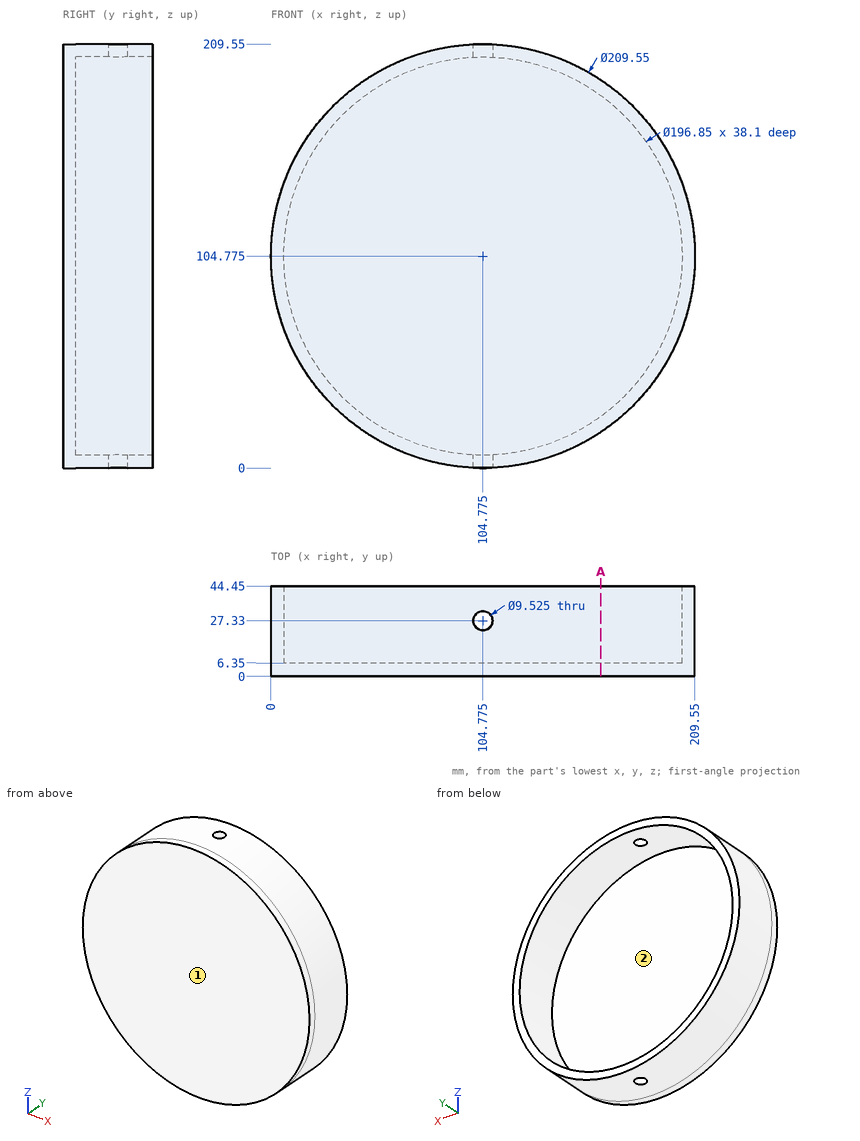
Part print with two shaded views. Sizes in mm from the minimum x, y, z corner. Give positions to 0.01 mm unless a question says otherwise; leave off trailing zeros. Order: outer loops, then holes, each group sorted by start corner. A loop starts at its lowest first (then second) coordinate and runs counter-clockwise, first axis right, second up. Notation, with made-up numbers: M -4.75,-21.75 L 11.25,-21.75 A14 cw 11.25,-9.75 Z; hole C 16.5,85.5 d10. An arc over 180 degrees is marked long. Write item = value, one per line.
Q1. Drill centre lines: line 1 (X direction, y = 26, z = 105); line 2 (Y direction, x = 145, z = 141); line 3 (Z direction, x = 31.5, y = 10.5) (1 decimal). Where is each one in solid material? Low to high. Write a range as [from, to].
Derived:
line_1 = [0, 6.35], [203.2, 209.55]
line_2 = [0, 6.35]
line_3 = [29.9, 39.1], [170.5, 179.7]
Q2. Two-plate mould, pull along X, no slides. Class the marked faces 1 and 2: pulls with the +X half, pulls with the -X half, needs draft (parallel to the pull), parting line crosses it, or undercut.
Derived:
face_1 = needs draft
face_2 = undercut
Q3. Flat gauge pins, fed straight in: pin 1 (2 mm diameter, centred on x = 73, y = 9, fed in from +Z); pin 2 (1.5 mm diameter, centred on x = 32.5, y = 25.5, fed in from +Z); pin 3 (7.5 mm diameter, centred on x = 104.78, y = 27.33, fed in from -Z); pin 4 (3 mm diameter, centred on x = 131.5, y = 4.5, fed in from +Z). Where does each tip first touch, or does it go through?
Derived:
pin_1 = 204.93
pin_2 = 181.34
pin_3 = through
pin_4 = 206.47
Q4. Cut at A-A, the plane x = 163. List the corners of the cut face in (y, z).
Derived:
outline = M 0,17.67 L 44.45,17.67 L 44.45,25.42 L 6.35,25.42 L 6.35,184.13 L 44.45,184.13 L 44.45,191.88 L 0,191.88 Z
